Geometry check sheet. Reference: the model listing, model coordinates, mm. Round coordinates to 2 decimals unless told otherwise and drop trailing zeros. Write each loop counter-clockwise with the first axis right and the second up, starting at its lowest first coordinate (ties: lowest second). Pieces come first, ordered by that corner, then holes. Notation, with made-up numbers: (-15.5, 30.25) -> (13.5, 30.25) arc R21 ccw to (13.5, 54.25) -> close; hole circle Ø6 at (0.25, 34.5). An arc over 180 degrees is marked (long way). Return JSON: item names as keys, results as strings. Group by question number.
from build123d import *

# Parameters (mm, degrees)
F0_W     = 2.54
F0_H     = 10.16
F1_DEPTH = 6.35


with BuildPart() as f1:
    # F0 (on Top) → F1 (new body)
    with BuildSketch(Plane.XY):
        with BuildLine():
            ThreePointArc((-36.84507, 47.773027), (-35.915134, 45.527963), (-33.67007, 44.598027))
            Line((-33.67007, 44.598027), (25.38493, 44.598027))
            ThreePointArc((25.38493, 44.598027), (27.629994, 45.527963), (28.55993, 47.773027))
            Line((28.55993, 47.773027), (28.55993, 154.732427))
            ThreePointArc((28.55993, 154.732427), (27.629994, 156.977491), (25.38493, 157.907427))
            Line((25.38493, 157.907427), (-33.67007, 157.907427))
            ThreePointArc((-33.67007, 157.907427), (-35.915134, 156.977491), (-36.84507, 154.732427))
            Line((-36.84507, 154.732427), (-36.84507, 47.773027))
        make_face()
        with Locations((-21.28757, 57.298027)):
            Rectangle(F0_W, F0_H, mode=Mode.SUBTRACT)
        with Locations((-21.28757, 82.698027)):
            Rectangle(F0_W, F0_H, mode=Mode.SUBTRACT)
        with Locations((13.00243, 57.298027)):
            Rectangle(F0_W, F0_H, mode=Mode.SUBTRACT)
        with Locations((13.00243, 82.698027)):
            Rectangle(F0_W, F0_H, mode=Mode.SUBTRACT)
        with Locations((-21.28757, 108.098027)):
            Rectangle(F0_W, F0_H, mode=Mode.SUBTRACT)
        with Locations((-21.28757, 133.498027)):
            Rectangle(F0_W, F0_H, mode=Mode.SUBTRACT)
        with Locations((13.00243, 108.098027)):
            Rectangle(F0_W, F0_H, mode=Mode.SUBTRACT)
        with Locations((13.00243, 133.498027)):
            Rectangle(F0_W, F0_H, mode=Mode.SUBTRACT)
    extrude(amount=F1_DEPTH)


solid = f1.part
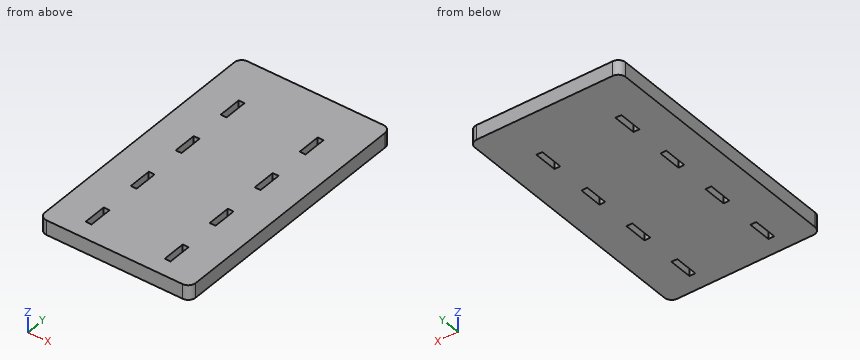
1) Material ranges on probe 1 along X at (y, z) = (105, 3.5), recorded low to high. Write a range as [from, to].
2) Sectioned sample at A-A on y = 83. Enter the section's corners in (x, z), and give its area (3 significant figures).
3) Sectioned sample at B-B on z = 1.5. State how many separate pieces and enclosed holes the cut face has, and give its area (3 significant figures).
Evaluation:
{
 "1": {"probe 1": "x = [-36.85, -22.56], [-20.02, 11.73], [14.27, 28.56]"},
 "2": {"outline": "(-36.85, 0) -> (-22.56, 0) -> (-22.56, 6.35) -> (-36.85, 6.35) -> close; (-20.02, 0) -> (11.73, 0) -> (11.73, 6.35) -> (-20.02, 6.35) -> close; (14.27, 0) -> (28.56, 0) -> (28.56, 6.35) -> (14.27, 6.35) -> close", "area": "383 mm2"},
 "3": {"separate pieces": "1", "enclosed holes": "8", "area": "7,200 mm2"}
}
